from build123d import *

# Parameters (mm, degrees)
F0_W     = 30
F0_H     = 30
F0_R     = 1.5
F0_R_2   = 4
F1_DEPTH = 2
F2_R     = 14.99999


# Not quite as in the source:
# - a fillet or chamfer is up to 0.001 mm smaller than in the source, because OpenCascade refuses the exact size


with BuildPart() as f1:
    # F0 (on Top) → F1 (new body)
    with BuildSketch(Plane.XY):
        with Locations((-15, 15)):
            Rectangle(F0_W, F0_H)
        with Locations((-4, 4)):
            Circle(F0_R, mode=Mode.SUBTRACT)
        with Locations((-16, 15)):
            Circle(F0_R_2, mode=Mode.SUBTRACT)
        with Locations((-4, 26)):
            Circle(F0_R, mode=Mode.SUBTRACT)
    extrude(amount=F1_DEPTH)

    # F2 (radius 15 in the source; OpenCascade refuses exactly that, so slightly less here)
    f2_edges = [f1.edges().sort_by_distance(p)[0] for p in [
        (-30, 0, 1),
        (-30, 30, 1),
    ]]
    fillet(f2_edges, radius=F2_R)


solid = f1.part
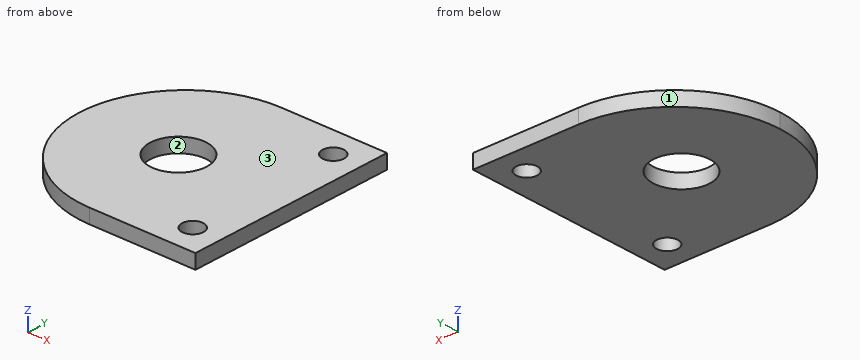
Geometry check sheet. Reference: the model listing, model coordinates, mm. Face numbers are marked on the shaded views. Give positions to 0.01 mm unless a question says otherwise; leave off trailing zeros. Order: outer loops, then holes, each group sorted by start corner. A loop starts at its lowest first (then second) coordinate and runs counter-clockwise, first axis right, second up.
1) Cross-section at B-B (z = 1). Give the number of separate pieces and of enclosed holes in the cut face, then the cut area to 3 significant figures.
Results are:
separate pieces: 1
enclosed holes: 3
area: 739 mm2
2) Gauge pin test, flat ends, axial feed: pin 1 (2.5 mm diameter, centred on x = -4, y = 26, fed in from +Z); pin 2 (1 mm diameter, centred on x = -17, z = 0.5, fed in from +Y). Record the tip position at first contact, or that the pin passes through.
Results are:
pin 1: passes through
pin 2: stops at y = 29.92
3) Cross-section at C-C (y = 26). Record the boundary of the cut face in (x, z).
Results are:
outline: (-25.2, 0) - (-5.5, 0) - (-5.5, 2) - (-25.2, 2) - close; (-2.5, 0) - (0, 0) - (0, 2) - (-2.5, 2) - close
4) Draft check along Y on the marked faces 1, 2 and 3. Enter one of: released by +Y, released by -Y, zero draft, split by the parting line, or undercut.
Results are:
face 1: released by +Y
face 2: undercut
face 3: zero draft
5) Material ranges on probe 1 along Y at (x, z) = (-4, 0.9); probe 2 along Y at (x, z) = (-3, 0.25); probe 3 along Y at (x, z) = (-16, 0.5), recorded low to high.
Results are:
probe 1: y = 0 to 2.5, 5.5 to 24.5, 27.5 to 30
probe 2: y = 0 to 2.88, 5.12 to 24.88, 27.12 to 30
probe 3: y = 0.03 to 11, 19 to 29.97
6) Cross-section at D-D (x = -13). Record the boundary of the cut face in (y, z).
Results are:
outline: (0, 0) - (12.35, 0) - (12.35, 2) - (0, 2) - close; (17.65, 0) - (30, 0) - (30, 2) - (17.65, 2) - close
7) Cross-section at A-A (x = -4). Record the boundary of the cut face in (y, z), then the cut area to 3 significant figures.
Results are:
outline: (0, 0) - (2.5, 0) - (2.5, 2) - (0, 2) - close; (5.5, 0) - (24.5, 0) - (24.5, 2) - (5.5, 2) - close; (27.5, 0) - (30, 0) - (30, 2) - (27.5, 2) - close
area: 48.0 mm2
